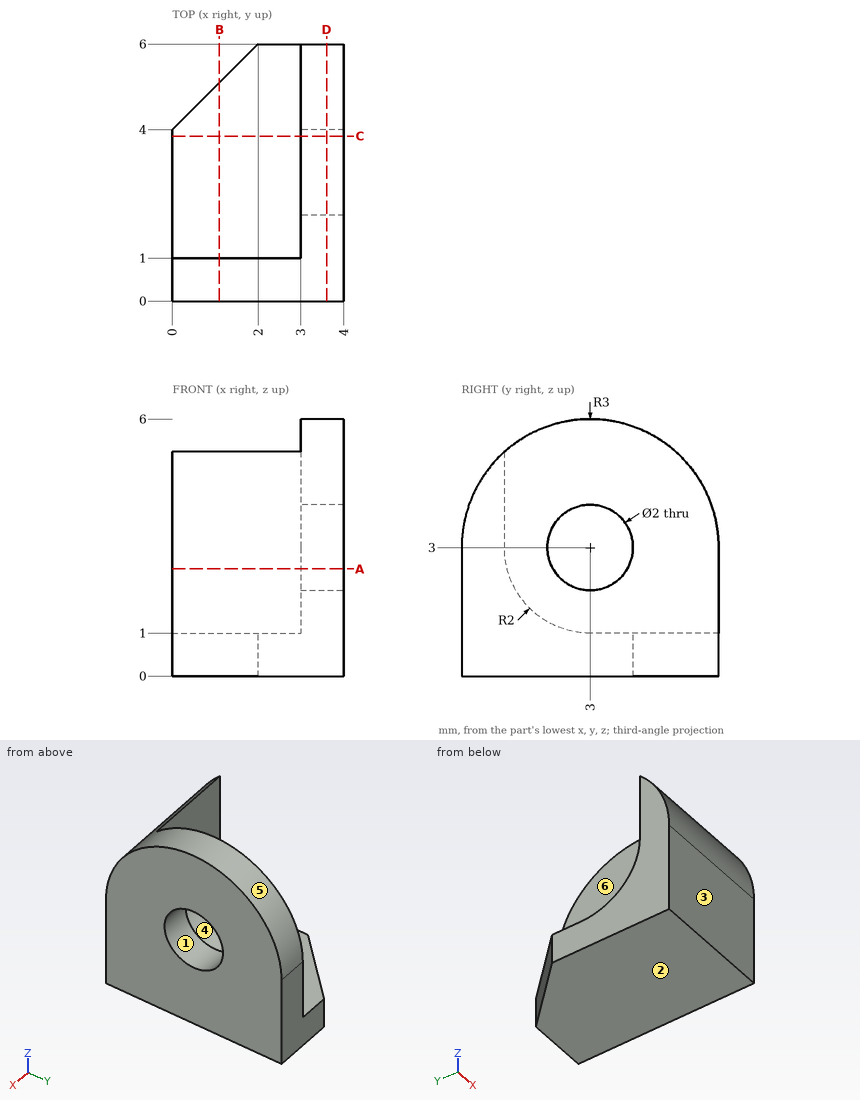
Study the drawing (mm; zero at the part's minimum x, y, z) and answer. A direction names the side the tool comes from. Give positions to 0.01 mm unless a question says otherwise; leave off trailing zeros. Loops run counter-clockwise (first coordinate to the right, second up) from the corner with the lowest first, then second, coordinate; pieces in that order, holes last. Notation, with made-up numbers: M -1.5,5 L 5.5,5 A15 cw 5.5,10 Z; hole C 30,13.25 d7. An arc over 180 degrees is marked long. One line per item, written item: value. Start each with the question number.
1. Which of the six approach directions +Z, -Z, +X, -X, +Y, -Y give full straight-line access (tool end or side, diameter ignored) to the marked faces 5 and 6?
2. Each of these flat-tipped pins is pushed along its axis until it touches: P1, Ø1.8, axis at x = 2, z = 4, coming from the +Y side; P2, Ø3, axis at y = 3, z = 3, coming from the -X side; P3, Ø2, axis at x = 3, y = 2.5, coming from the -Z side. Where does it stop, or does it pass through?
3. Find the intervals of material crossed by probe 1 along Y at (x, z) = (3.45, 3); probe 2 along X at (y, z) = (3.9, 5.7), in increasing order.
4. Determine the mould class of the marked faces 1, 2, 3 and 4 for opening direction Z: released by +Z, released by -Z, zero draft, split by the parting line, or undercut.
5. Find section B-B (x = 1.1). Give the vertices of the cut face in (y, z).
6. Find section C-C (y = 3.85). Give the vertices of the cut face in (x, z).
7. Find section A-A (z = 2.5). Give the vertices of the cut face in (x, y), and give its area (3 significant figures).
8. Find section D-D (x = 3.6). Give the vertices of the cut face in (y, z), and give its area (3 significant figures).
Reported:
1. face 5: +Z, +X, -X
1. face 6: +Z, -X, +Y
2. P1: stops at y = 1
2. P2: stops at x = 3
2. P3: stops at z = 0
3. probe 1: y = 0 to 2, 4 to 6
3. probe 2: x = 3 to 4
4. face 1: undercut
4. face 2: released by -Z
4. face 3: zero draft
4. face 4: released by +Z
5. outline: M 0,0 L 5.1,0 L 5.1,1 L 3,1 A2 cw 1,3 L 1,5.24 A3 ccw 0,3 Z
6. outline: M 0,0 L 4,0 L 4,2.47 L 3,2.47 L 3,1 L 0,1 Z; M 3,3.53 L 4,3.53 L 4,5.88 L 3,5.88 Z
7. outline: M 0,0 L 4,0 L 4,2.13 L 3,2.13 L 3,1.06 L 0,1.06 Z; M 3,3.87 L 4,3.87 L 4,6 L 3,6 Z
7. area: 7.46 mm²
8. outline: M 0,0 L 6,0 L 6,3 A3 ccw 0,3 Z; hole C 3,3 d2
8. area: 29.0 mm²
